from build123d import *

# Parameters (mm, degrees)
F1_DEPTH = 25.4
F3_DEPTH = 12.701
F5_DEPTH = 12.701
F7_DEPTH = 12.701


with BuildPart() as f1:
    # F0 (on Front) → F1 (new body)
    with BuildSketch(Plane.XZ):
        Polygon((0, 50.8), (0, 0), (57.15, 0), (57.15, 12.7), (12.7, 12.7), (12.7, 50.8), align=None)
    extrude(amount=F1_DEPTH)

    # F2 (on face) → F3 (cut, through all)
    with BuildSketch(Plane.YZ.offset(12.7)):
        with BuildLine():
            ThreePointArc((-6.35, 31.75), (-12.7, 38.1), (-19.05, 31.75))
            Line((-19.05, 31.75), (-6.35, 31.75))
        make_face()
        with BuildLine():
            Line((-6.35, 31.75), (-19.05, 31.75))
            ThreePointArc((-19.05, 31.75), (-12.7, 25.4), (-6.35, 31.75))
        make_face()
        with BuildLine():
            Line((-19.05, 50.8), (-19.05, 31.75))
            ThreePointArc((-19.05, 31.75), (-12.7, 38.1), (-6.35, 31.75))
            Line((-6.35, 31.75), (-6.35, 50.8))
            Line((-6.35, 50.8), (-19.05, 50.8))
        make_face()
    extrude(amount=-F3_DEPTH, mode=Mode.SUBTRACT)

    # F4 (on face) → F5 (cut, through all)
    with BuildSketch(Plane.YZ.offset(12.7)):
        with BuildLine():
            Line((-25.4, 50.8), (-25.4, 38.3654093824))
            ThreePointArc((-25.4, 38.3654093824), (-23.6656953438, 44.6406010825), (-19.05, 49.2320278765))
            Line((-19.05, 49.2320278765), (-19.05, 50.8))
            Line((-19.05, 50.8), (-25.4, 50.8))
        make_face()
        with BuildLine():
            Line((-6.35, 50.8), (-6.35, 49.2320278765))
            ThreePointArc((-6.35, 49.2320278765), (-1.7343046562, 44.6406010825), (0, 38.3654093824))
            Line((0, 38.3654093824), (0, 50.8))
            Line((0, 50.8), (-6.35, 50.8))
        make_face()
    extrude(amount=-F5_DEPTH, mode=Mode.SUBTRACT)

    # F6 (on face) → F7 (cut, through all)
    with BuildSketch(Plane.XY.offset(12.7)):
        with BuildLine():
            ThreePointArc((25.4, -6.35), (19.05, -12.7), (25.4, -19.05))
            Line((25.4, -19.05), (25.4, -6.35))
        make_face()
        with BuildLine():
            Line((25.4, -6.35), (25.4, -19.05))
            ThreePointArc((25.4, -19.05), (29.8901280605, -17.1901280605), (31.75, -12.7))
            ThreePointArc((31.75, -12.7), (29.8901280605, -8.2098719395), (25.4, -6.35))
        make_face()
        with BuildLine():
            ThreePointArc((44.45, -6.35), (38.1, -12.7), (44.45, -19.05))
            Line((44.45, -19.05), (44.45, -6.35))
        make_face()
        with BuildLine():
            Line((44.45, -6.35), (44.45, -19.05))
            ThreePointArc((44.45, -19.05), (48.9401280605, -17.1901280605), (50.8, -12.7))
            ThreePointArc((50.8, -12.7), (48.9401280605, -8.2098719395), (44.45, -6.35))
        make_face()
        with BuildLine():
            ThreePointArc((57.15, -12.7), (53.4302561211, -21.6802561211), (44.45, -25.4))
            Line((44.45, -25.4), (57.15, -25.4))
            Line((57.15, -25.4), (57.15, -12.7))
        make_face()
        with BuildLine():
            ThreePointArc((44.45, 0), (53.4302561211, -3.7197438789), (57.15, -12.7))
            Line((57.15, -12.7), (57.15, 0))
            Line((57.15, 0), (44.45, 0))
        make_face()
    extrude(amount=-F7_DEPTH, mode=Mode.SUBTRACT)


solid = f1.part
Input: part model. Units: mm. Frame: model coordinates. A direction names the side the tool comes from. Coordinates: 2 decimals unless noted, no trailing zeros. Write each loop counter-clockwise with the first axis right and the second up, starting at its lowest first coordinate (ties: lowest second). Pieces come first, ordered by that corner, then holes. Notation, with made-up numbers: M 7,-5 L 25,-5 A8 cw 25,10 Z; hole C 29.25,20.25 d9. An arc over 180 degrees is marked long. Answer as a JSON object with one key per item and string values. Group by question number.
(1) Ray query, line 1 along X through (y, z) = (-17.75, 19.5); line 2 along Y through (x, z) = (9.5, 47). Return the intervals inside material, ascending. Write a range as [from, to].
(2) Contact query for flat-ended pins moving along their axis: P1, Ø10, axis at y = -4, z = 42.5, coming from the +X side; P2, Ø3, axis at x = 20, y = -6, coming from the +Z side; P3, Ø6, axis at x = 9.5, y = -11.5, coming from the +Z side. Output: stop coordinate, or through.
(3) Section B-B on x = 4. Output: boundary loops of the cut face in (y, z), plus the area to 3 significant figures.
(4) Section A-A on y = -14.25. Output: boundary loops of the cut face in (x, z), plus the area to 3 significant figures.
(5) Section C-C on x = 42.5. Output: boundary loops of the cut face in (y, z), plus the area to 3 significant figures.
(6) Section D-D on y = -23.75. Output: boundary loops of the cut face in (x, z), plus the area to 3 significant figures.
(7) Mould query, pull axis Y, two halves, no side actions, for faces 4 (the face through (6.44, -1.78, 44.72)), 5 (the face through (6, -19.05, 41)), 6 (the face through (22, -7, 0)). Classes: pulls with the +Y half, pulls with the -Y half, needs draft (parallel to the pull), parting line crosses it, or undercut.
(8) Set-up query: faces 1 (the face through (12.7, -13, 23)), 2 (the face through (0, -13, 19)), 3 (the face through (6, -6.35, 40)). Return all of +Z, -Z, +X, -X, +Y, -Y with unobstructed straight access to the full face (end or side cutting, diameter ignored); none if empty.
Result set:
{
 "1": {"line 1": "x = [0, 12.7]", "line 2": "y = [-21.89, -19.05], [-6.35, -3.51]"},
 "2": {"P1": "stops at x = 12.7", "P2": "stops at z = 12.7", "P3": "stops at z = 26.99"},
 "3": {"outline": "M -25.4,0 L 0,0 L 0,38.37 A12.7 ccw -6.35,49.23 L -6.35,31.75 A6.35 cw -19.05,31.75 L -19.05,49.23 A12.7 ccw -25.4,38.37 Z", "area": "925 mm2"},
 "4": {"outline": "M 0,0 L 19.24,0 L 19.24,12.7 L 12.7,12.7 L 12.7,25.59 L 0,25.59 Z; M 31.56,0 L 38.29,0 L 38.29,12.7 L 31.56,12.7 Z; M 50.61,0 L 57.06,0 L 57.06,12.7 L 50.61,12.7 Z", "area": "576 mm2"},
 "5": {"outline": "M -25.4,0 L -18.74,0 L -18.74,12.7 L -25.4,12.7 Z; M -6.66,0 L 0,0 L 0,12.7 L -6.66,12.7 Z", "area": "169 mm2"},
 "6": {"outline": "M 0,0 L 50.71,0 L 50.71,12.7 L 12.7,12.7 L 12.7,44.49 L 0,44.49 Z", "area": "1,050 mm2"},
 "7": {"face 4": "pulls with the +Y half", "face 5": "undercut", "face 6": "needs draft"},
 "8": {"face 1": "+Z, +X, +Y, -Y", "face 2": "+Z, -Z, -X, +Y, -Y", "face 3": "+Z, +X, -X"}
}
